from build123d import *

# Parameters (mm, degrees)
SKETCH_1_W          = 60
SKETCH_1_H          = 50
SKETCH_1_R          = 15
EXTRUDE_5_DEPTH     = 5
SKETCH_4_W          = 60
SKETCH_4_H          = 50
SKETCH_4_R          = 5.5
EXTRUDE_6_DEPTH     = 5
SKETCH_5_R          = 1.6
CUT_EXTRUDE_1_DEPTH = 10
SKETCH_6_W          = 60
SKETCH_6_H          = 10
EXTRUDE_7_DEPTH     = 7
FILLET_3_R          = 10
FILLET_5_R          = 10
FILLET_6_R          = 5
FILLET_7_R          = 5
SKETCH_8_R          = 41.984876442
CUT_EXTRUDE_3_DEPTH = 3
SKETCH_7_R          = 4
CUT_EXTRUDE_4_DEPTH = 3
SKETCH_9_R          = 15
EXTRUDE_8_DEPTH     = 7
SKETCH_10_R         = 15
CUT_EXTRUDE_5_DEPTH = 2
SKETCH_11_R         = 5.5
CUT_EXTRUDE_6_DEPTH = 45.147480109


with BuildPart() as part:
    # 草图1 → 凸台-拉伸5 (new body)
    with BuildSketch(Plane.XY):
        Rectangle(SKETCH_1_W, SKETCH_1_H)
        Circle(SKETCH_1_R, mode=Mode.SUBTRACT)
    extrude(amount=EXTRUDE_5_DEPTH)

    # 草图4 → 凸台-拉伸6 (add)
    with BuildSketch(Plane.XY.offset(5)):
        Rectangle(SKETCH_4_W, SKETCH_4_H)
        Circle(SKETCH_4_R, mode=Mode.SUBTRACT)
    extrude(amount=EXTRUDE_6_DEPTH)

    # 草图5 → 切除-拉伸1 (cut)
    with BuildSketch(Plane(origin=(0, 0, 0), x_dir=(-1, 0, 0), z_dir=(0, 0, -1))):
        with Locations((-20, 22)):
            Circle(SKETCH_5_R)
        with Locations((-25, -18)):
            Circle(SKETCH_5_R)
        with Locations((20, 22)):
            Circle(SKETCH_5_R)
        with Locations((25, -18)):
            Circle(SKETCH_5_R)
    extrude(amount=-CUT_EXTRUDE_1_DEPTH, mode=Mode.SUBTRACT)

    # 草图6 → 凸台-拉伸7 (add)
    with BuildSketch(Plane(origin=(0, 25, 0), x_dir=(1, 0, 0), z_dir=(0, 1, 0))):
        with Locations((0, -5)):
            Rectangle(SKETCH_6_W, SKETCH_6_H)
    extrude(amount=EXTRUDE_7_DEPTH)

    # 圆角3
    fillet_3_edges = [part.edges().sort_by_distance(p)[0] for p in [
        (-30, 32, 5),
    ]]
    fillet(fillet_3_edges, radius=FILLET_3_R)

    # 圆角5
    fillet_5_edges = [part.edges().sort_by_distance(p)[0] for p in [
        (30, 32, 5),
    ]]
    fillet(fillet_5_edges, radius=FILLET_5_R)

    # 圆角6
    fillet_6_edges = [part.edges().sort_by_distance(p)[0] for p in [
        (-30, -25, 5),
    ]]
    fillet(fillet_6_edges, radius=FILLET_6_R)

    # 圆角7
    fillet_7_edges = [part.edges().sort_by_distance(p)[0] for p in [
        (30, -25, 5),
    ]]
    fillet(fillet_7_edges, radius=FILLET_7_R)

    # 草图8 → 切除-拉伸3 (cut)
    with BuildSketch(Plane(origin=(0, 0, 0), x_dir=(-1, 0, 0), z_dir=(0, 0, -1))):
        Circle(SKETCH_8_R)
    extrude(amount=-CUT_EXTRUDE_3_DEPTH, mode=Mode.SUBTRACT)

    # 草图7 → 切除-拉伸4 (cut)
    with BuildSketch(Plane.XY.offset(10)):
        with Locations((-20, 22)):
            Circle(SKETCH_7_R)
        with Locations((20, 22)):
            Circle(SKETCH_7_R)
        with Locations((-25, -18)):
            Circle(SKETCH_7_R)
        with Locations((25, -18)):
            Circle(SKETCH_7_R)
    extrude(amount=-CUT_EXTRUDE_4_DEPTH, mode=Mode.SUBTRACT)

    # 草图9 → 凸台-拉伸8 (add)
    with BuildSketch(Plane(origin=(0, 0, 3), x_dir=(-1, 0, 0), z_dir=(0, 0, -1))):
        Circle(SKETCH_9_R)
    extrude(amount=-EXTRUDE_8_DEPTH)

    # 草图10 → 切除-拉伸5 (cut)
    with BuildSketch(Plane(origin=(0, 0, 3), x_dir=(-1, 0, 0), z_dir=(0, 0, -1))):
        with Locations((0, 14)):
            Circle(SKETCH_10_R)
    extrude(amount=-CUT_EXTRUDE_5_DEPTH, mode=Mode.SUBTRACT)

    # 草图11 → 切除-拉伸6 (cut, through all)
    with BuildSketch(Plane(origin=(0, 0, 5), x_dir=(-1, 0, 0), z_dir=(0, 0, -1))):
        with Locations((0, 14)):
            Circle(SKETCH_11_R)
    extrude(amount=-CUT_EXTRUDE_6_DEPTH, mode=Mode.SUBTRACT)


solid = part.part
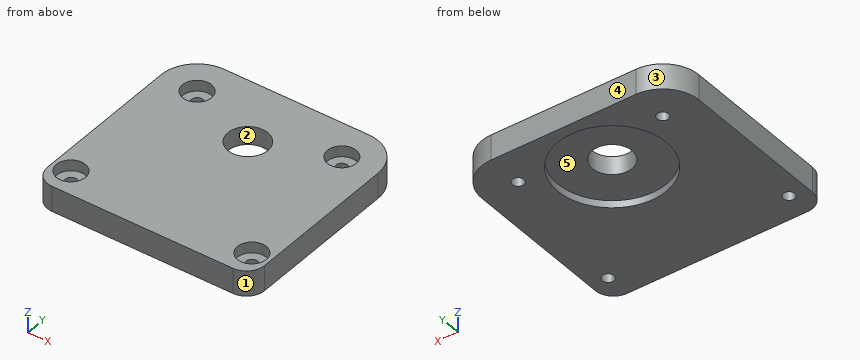
Check sheet for the modelled part. Datum: model origin and axes. Units: mm. Face numbers are marked on the shaded views. A direction names the side the tool comes from. Give positions to 0.01 mm unless a question says otherwise; leave off trailing zeros. Loops run counter-clockwise (first coordinate to the right, second up) from the corner with the lowest first, then second, coordinate; pieces in that order, holes last. Notation, with made-up numbers: M 88.5,48.25 L 98.5,48.25 A19 ccw 98.5,81.25 Z; hole C 66,-17 d1. An arc over 180 degrees is marked long. Return JSON: item names as keys, results as strings. Group by question number.
1. Cross-section at C-C on z = 7.75. Record the boundary of the cut face in (x, y), plus the area to 3 significant figures.
2. Mould release check, pull along X, two halves, no side actions. Record for the marked faces 1, 2 and 3: released by +X, released by -X, zero draft, split by the parting line, or undercut.
3. Tool access check on the marked faces 4 and 5. Record the directions out of +Z, -Z, +X, -X, +Y, -Y that give a thin tool (end or side, any length) a straight path to the whole face; none if there is none.
4. Cross-section at A-A on y = -18. Record the boundary of the cut face in (x, z).
5. Cross-section at B-B on x = 0. Record the boundary of the cut face in (y, z), plus the area to 3 significant figures.
6. Go/stop test with flat-tipped pins: pin 1 (4 mm diameter, centred on x = 21.5, y = 22.5, fed in from +Z); pin 2 (2.5 mm diameter, centred on x = -20, y = 22, fed in from -Z). Record where each tip stops, or that it passes through.
7. Thickness scan on L1, parallel to X at y = 24.5, z = 9; L2, parallel to Y at x = 22.5, z = 9.5; L3, parallel to Y at x = 21.5, z = 8.25. Record the ranges inside material, lowest first.
8. Cross-section at D-D on y = 13. Record the boundary of the cut face in (x, z), plus the area to 3 significant figures.
Return value:
{
 "1": {"outline": "M -30,-20 A5 ccw -25,-25 L 25,-25 A5 ccw 30,-20 L 30,22 A10 ccw 20,32 L -20,32 A10 ccw -30,22 Z; hole C -25,-18 d8; hole C -20,22 d8; hole C 0,14 d11; hole C 20,22 d8; hole C 25,-18 d8", "area": "3,070 mm^2"},
 "2": {"face 1": "released by +X", "face 2": "undercut", "face 3": "released by -X"},
 "3": {"face 4": "+Z, -Z, +X, -X, +Y", "face 5": "-Z"},
 "4": {"outline": "M -30,3 L -26.6,3 L -26.6,7 L -29,7 L -29,10 L -30,10 Z; M -23.4,3 L 23.4,3 L 23.4,7 L 21,7 L 21,10 L -21,10 L -21,7 L -23.4,7 Z; M 26.6,3 L 30,3 L 30,10 L 29,10 L 29,7 L 26.6,7 Z"},
 "5": {"outline": "M -25,3 L -1,3 L -1,5 L 8.5,5 L 8.5,10 L -25,10 Z; M 19.5,5 L 29,5 L 29,3 L 32,3 L 32,10 L 19.5,10 Z", "area": "284 mm^2"},
 "6": {"pin 1": "z = 7", "pin 2": "through"},
 "7": {"L1": "-29.68 to -23.12, -16.88 to 16.88, 23.12 to 29.68", "L2": "-25 to -21.12, -14.88 to 18.88, 25.12 to 31.68", "L3": "-25 to -19.94, -16.06 to 18.29, 25.71 to 31.89"},
 "8": {"outline": "M -30,3 L -14.97,3 L -14.97,5 L -5.41,5 L -5.41,10 L -30,10 Z; M 5.41,5 L 14.97,5 L 14.97,3 L 30,3 L 30,10 L 5.41,10 Z", "area": "306 mm^2"}
}
